```python
from build123d import *

# Parameters (mm, degrees)
SKETCH1_W          = 5.564434946
SKETCH1_H          = 300
CUT_EXTRUDE1_DEPTH = 5.9
CUT_EXTRUDE2_DEPTH = 5.9
HOLE1_D            = 4.92
HOLE1_DEPTH        = 10.5
HOLE1_TIP          = 1.420281662
CHAMFER2_SIZE      = 0.54


with BuildPart() as part:
    # Sketch1 → Revolve1 (revolve)
    with BuildSketch(Plane.XZ, mode=Mode.PRIVATE) as revolve1_sk:
        with Locations((2.782217473, -144.435565054)):
            Rectangle(SKETCH1_W, SKETCH1_H)
    revolve(revolve1_sk.sketch.rotate(Axis((0, 0, 5.564434946), (0, 0, -1)), 180), axis=Axis((0, 0, 5.564434946), (0, 0, -1)))

    # Sketch2 → Cut-Extrude1 (cut)
    with BuildSketch(Plane.XY.offset(5.564434946)):
        with BuildLine():
            Line((-5, -3.31662479), (-5, 3.31662479))
            ThreePointArc((-5, 3.31662479), (-6, 0), (-5, -3.31662479))
        make_face()
    extrude(amount=-CUT_EXTRUDE1_DEPTH, mode=Mode.SUBTRACT)

    # Sketch3 → Cut-Extrude2 (cut)
    with BuildSketch(Plane.XY.offset(5.564434946)):
        with BuildLine():
            Line((5, 3.31662479), (5, -3.31662479))
            ThreePointArc((5, -3.31662479), (6, 0), (5, 3.31662479))
        make_face()
    extrude(amount=-CUT_EXTRUDE2_DEPTH, mode=Mode.SUBTRACT)

    # Hole1
    with Locations(Plane.XY.offset(5.564434946)):
        with Locations((0, 0)):
            Hole(HOLE1_D / 2, depth=HOLE1_DEPTH)
            with Locations((0, 0, -(HOLE1_DEPTH + HOLE1_TIP / 2))):  # 120° drill point
                Cone(0, HOLE1_D / 2, HOLE1_TIP, mode=Mode.SUBTRACT)

    # Chamfer2
    chamfer2_edges = [part.edges().sort_by_distance(p)[0] for p in [
        (2.46, 0, 5.564434946),
    ]]
    chamfer(chamfer2_edges, length=CHAMFER2_SIZE)


solid = part.part
```
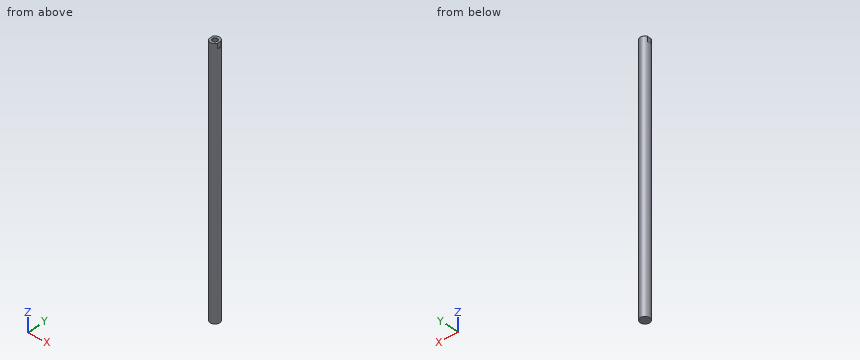
Geometry check sheet. Reference: the model listing, model coordinates, mm. Round coordinates to 2 decimals unless told otherwise and drop trailing zeros. Write each loop counter-clockwise with the first axis right and the second up, starting at its lowest first coordinate (ties: lowest second). Pieces come first, ordered by that corner, then holes. Notation, with made-up numbers: (61, 12) -> (81, 12) arc R20 cw to (81, 45) -> close; hole circle Ø6 at (38, 74.5). An arc over 180 degrees is marked (long way). Put each result on its own line as item: value.
1) Thickness scan on probe 1 along X at (y, z) = (0, 1); probe 2 along X at (y, z) = (0, -2.5). Record the ranges inside material, lowest first. Write a range as from..to.
Recorded:
probe 1: x = -5..-2.46, 2.46..5
probe 2: x = -5.56..-2.46, 2.46..5.56
2) Depth check by flat-ended pin: P1, Ø1, axis at y = -1, z = -50.5, coming from the +X side; P2, Ø2.5, axis at y = 0, z = 1.5, coming from the -X side; P3, Ø1, axis at y = 2.5, z = -59.5, coming from the +X side. Enter the tip coordinate at first touch or a pass-through.
Recorded:
P1: stops at x = 5.54
P2: stops at x = -5
P3: stops at x = 5.19
3) Cross-section at A-A, the plane z = -32. Enter the section's corners in (x, y).
Recorded:
outline: circle Ø11.13 at (0, 0)
